Can you work these out from the model? Positions are in its coordinate system, mm. Coordinates: 2 decimals unless noted, no trailing zeros. Loops run counter-clockwise (first coordinate to the right, second up) from the corner with the lowest first, then second, coordinate; pieces in that order, holes last. Notation, with made-up numbers: M -13.5,-11 L 34.5,-11 A15 cw 34.5,13 Z; hole C 8,-31 d1. An arc over 180 degrees is marked long. Answer as a JSON object with one key per item and string values. Group by question number.
Item 1: I'm going to push flat-ended pins straight in: pin 1 Ø1 at (y, z) = (1.5, 158.5) entering from +X; pin 2 Ø1.7 at (x, z) = (-0.5, 106) entering from -Y. Where does each tip first touch, or does it pass through?
Item 2: Suppose I cut it at C-C (x = -0.25). Write out the boundary of the cut face in (y, z).
Item 3: If I drill on line 1 (X direction, y = 1.3, z = 420.5); line 2 (X direction, y = 0.6, z = 264.5); line 3 (Y direction, x = 1, z = 777), over which ranges is the centre line in solid material (lowest first)?
Item 4: Suppose I cut it at B-B (y = 1.05). Write out the boundary of the cut face in (x, z).
Item 5: Suppose I cut it at A-A (z = -365.5). Write out the boundary of the cut face in (x, y), then the cut area to 3 significant figures.
```python
from build123d import *

# Parameters (mm, degrees)
BOSS_EXTRUDE1_DEPTH      = 1000
BOSS_EXTRUDE1_DEPTH_BACK = 1000


with BuildPart() as part:
    # Sketch1 → Boss-Extrude1 (new body, two sides)
    with BuildSketch(Plane.XY) as boss_extrude1_sk:
        with BuildLine():
            Line((-3.6, 3.35), (-3, 0))
            Line((-3, 0), (-2.2, 0))
            Line((-2.2, 0), (-2.735217071, 2.988295315))
            ThreePointArc((-2.735217071, 2.988295315), (-2.659117427, 3.274614514), (-2.390699246, 3.4))
            Line((-2.390699246, 3.4), (-2.2, 3.4))
            Line((-2.2, 3.4), (-2.070472639, 4.88050451))
            ThreePointArc((-2.070472639, 4.88050451), (-1.958261067, 5.108047068), (-1.721804495, 5.2))
            Line((-1.721804495, 5.2), (1.721804495, 5.2))
            ThreePointArc((1.721804495, 5.2), (1.958261067, 5.108047068), (2.070472639, 4.88050451))
            Line((2.070472639, 4.88050451), (2.2, 3.4))
            Line((2.2, 3.4), (2.390699246, 3.4))
            ThreePointArc((2.390699246, 3.4), (2.659117427, 3.274614514), (2.735217071, 2.988295315))
            Line((2.735217071, 2.988295315), (2.2, 0))
            Line((2.2, 0), (3, 0))
            Line((3, 0), (3.6, 3.35))
            ThreePointArc((3.6, 3.35), (3.497487373, 3.597487373), (3.25, 3.7))
            Line((3.25, 3.7), (3, 3.7))
            Line((3, 3.7), (2.835477174, 5.58050451))
            ThreePointArc((2.835477174, 5.58050451), (2.723265602, 5.808047068), (2.486809029, 5.9))
            Line((2.486809029, 5.9), (-2.486809029, 5.9))
            ThreePointArc((-2.486809029, 5.9), (-2.723265602, 5.808047068), (-2.835477174, 5.58050451))
            Line((-2.835477174, 5.58050451), (-3, 3.7))
            Line((-3, 3.7), (-3.25, 3.7))
            ThreePointArc((-3.25, 3.7), (-3.497487373, 3.597487373), (-3.6, 3.35))
        make_face()
    extrude(amount=BOSS_EXTRUDE1_DEPTH)
    extrude(boss_extrude1_sk.sketch, amount=-BOSS_EXTRUDE1_DEPTH_BACK)


solid = part.part
```
From the geometry:
{
 "1": {"pin 1": "x = 3.36", "pin 2": "y = 5.2"},
 "2": {"outline": "M 5.2,-1000 L 5.9,-1000 L 5.9,1000 L 5.2,1000 Z"},
 "3": {"line 1": "-3.23 to -2.43, 2.43 to 3.23", "line 2": "-3.11 to -2.31, 2.31 to 3.11", "line 3": "5.2 to 5.9"},
 "4": {"outline": "M -3.19,-1000 L -2.39,-1000 L -2.39,1000 L -3.19,1000 Z; M 2.39,-1000 L 3.19,-1000 L 3.19,1000 L 2.39,1000 Z"},
 "5": {"outline": "M -3.6,3.35 L -3,0 L -2.2,0 L -2.74,2.99 A0.35 cw -2.39,3.4 L -2.2,3.4 L -2.07,4.88 A0.35 cw -1.72,5.2 L 1.72,5.2 A0.35 cw 2.07,4.88 L 2.2,3.4 L 2.39,3.4 A0.35 cw 2.74,2.99 L 2.2,0 L 3,0 L 3.6,3.35 A0.35 ccw 3.25,3.7 L 3,3.7 L 2.84,5.58 A0.35 ccw 2.49,5.9 L -2.49,5.9 A0.35 ccw -2.84,5.58 L -3,3.7 L -3.25,3.7 A0.35 ccw Z", "area": "12.8 mm2"}
}
